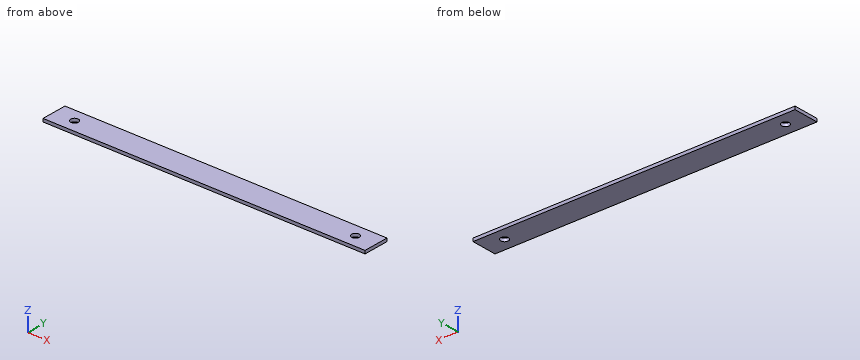
from build123d import *

# Parameters (mm, degrees)
SKETCH1_W           = 125
SKETCH1_H           = 10
BOSS_EXTRUDE1_DEPTH = 1.2
SKETCH2_R           = 1.5
CUT_EXTRUDE1_DEPTH  = 5


with BuildPart() as part:
    # Sketch1 → Boss-Extrude1 (new body)
    with BuildSketch(Plane.XY):
        with Locations((62.5, 5)):
            Rectangle(SKETCH1_W, SKETCH1_H)
    extrude(amount=BOSS_EXTRUDE1_DEPTH)

    # Sketch2 → Cut-Extrude1 (cut, symmetric)
    with BuildSketch(Plane.XY):
        with Locations((8, 5)):
            Circle(SKETCH2_R)
        with Locations((117, 5)):
            Circle(SKETCH2_R)
    extrude(amount=CUT_EXTRUDE1_DEPTH, both=True, mode=Mode.SUBTRACT)


solid = part.part
The listing builds one solid part. Answer for the finished solid, in the listing's coordinates (mm). Give positions to 0.01 mm unless a question says otherwise; leave off trailing zeros. Order: outer loops, then holes, each group sorted by start corner. A loop starts at its lowest first (then second) coordinate and runs counter-clockwise, first axis right, second up. Notation, with made-up numbers: (53.5, 12.25) - (108.5, 12.25) arc R22 cw to (108.5, 20.25) - close; hole circle Ø6 at (9.5, -16). An arc over 180 degrees is marked (long way). One line per item, written item: value. Start each with the question number.
1) A cutting plane is placed at B-B on x = 117. Give the vertices of the cut face in (y, z).
2) Given pin 1 Ø2.5 at (x, y) = (8, 5) entering from -Z, flat-ended and moving along its own axis, determine where the tip first touches the part or whether it passes through.
3) A cutting plane is placed at A-A on y = 5. Give the vertices of the cut face in (x, z), then the cut area to 3 significant figures.
4) Find the intervals of material crossed by L1, parallel to Y at x = 117, z = 0.9; L2, parallel to X at y = 4.5, z = 0.6, in increasing order.
Answer sheet:
1. outline: (0, 0) - (3.5, 0) - (3.5, 1.2) - (0, 1.2) - close; (6.5, 0) - (10, 0) - (10, 1.2) - (6.5, 1.2) - close
2. pin 1: passes through
3. outline: (0, 0) - (6.5, 0) - (6.5, 1.2) - (0, 1.2) - close; (9.5, 0) - (115.5, 0) - (115.5, 1.2) - (9.5, 1.2) - close; (118.5, 0) - (125, 0) - (125, 1.2) - (118.5, 1.2) - close
3. area: 143 mm2
4. L1: y = 0 to 3.5, 6.5 to 10
4. L2: x = 0 to 6.59, 9.41 to 115.59, 118.41 to 125
